Source: three-view drawing plus pictorial views. Frame: mm from the lowest corner of the part. Give positions to 0.01 mm unless a question says otherwise; leave off trailing zeros. Loops run counter-clockwise (first coordinate to the right, second up) from the corner with the lowest first, then second, coordinate; pieces in that order, holes last. Notation, with made-up numbers: M 51.5,23 L 94.5,23 A29 cw 94.5,60 Z; hole C -20,83.5 d11. An arc over 180 degrees is marked long. One line per item, written item: value. Start each with the question number.
(1) Section A-A on x = 3.81. Output: boundary loops of the cut face in (y, z).
(2) Section B-B on y = 3.81. Output: boundary loops of the cut face in (x, z).
(3) Ray query, line 1 along Y through (x, z) = (3.81, 1.05); line 2 along X through (y, z) = (72.39, 0.7); line 3 along Y through (x, z) = (5, 1). Return the intervals inside material, ascending. Write a range as from..to.
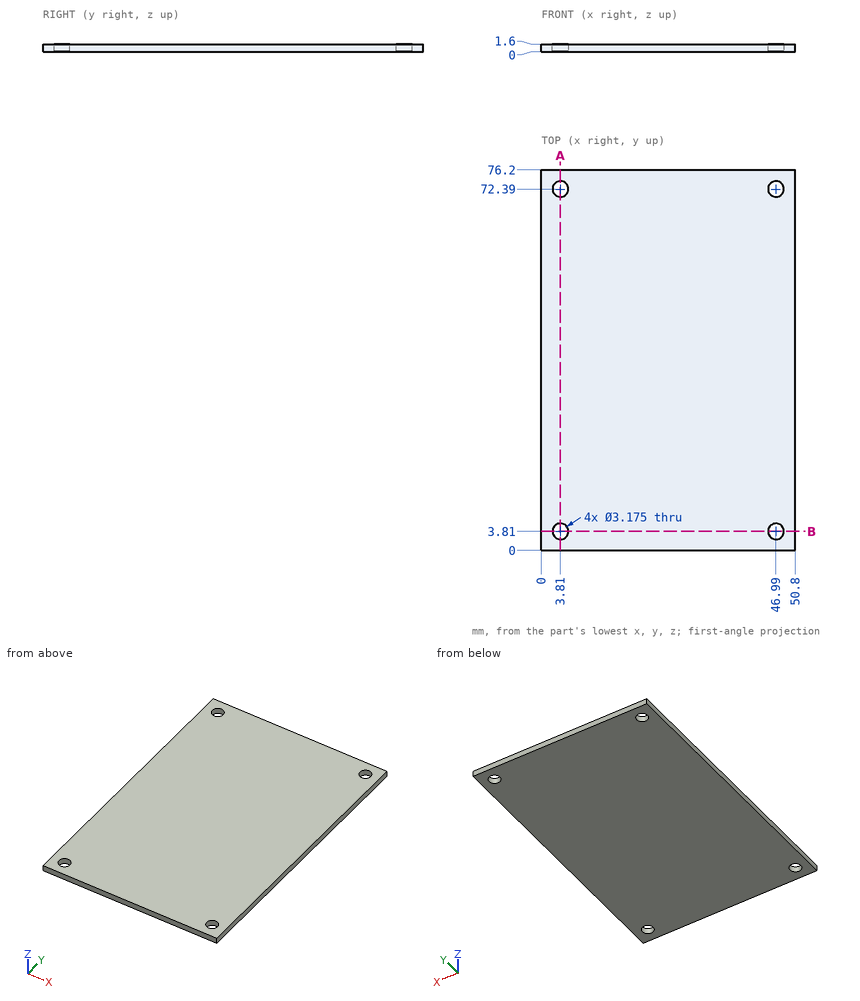
Output values:
1. outline: M 0,0 L 2.22,0 L 2.22,1.6 L 0,1.6 Z; M 5.4,0 L 70.8,0 L 70.8,1.6 L 5.4,1.6 Z; M 73.98,0 L 76.2,0 L 76.2,1.6 L 73.98,1.6 Z
2. outline: M 0,0 L 2.22,0 L 2.22,1.6 L 0,1.6 Z; M 5.4,0 L 45.4,0 L 45.4,1.6 L 5.4,1.6 Z; M 48.58,0 L 50.8,0 L 50.8,1.6 L 48.58,1.6 Z
3. line 1: y = 0..2.22, 5.4..70.8, 73.98..76.2
3. line 2: x = 0..2.22, 5.4..45.4, 48.58..50.8
3. line 3: y = 0..2.76, 4.86..71.34, 73.44..76.2
